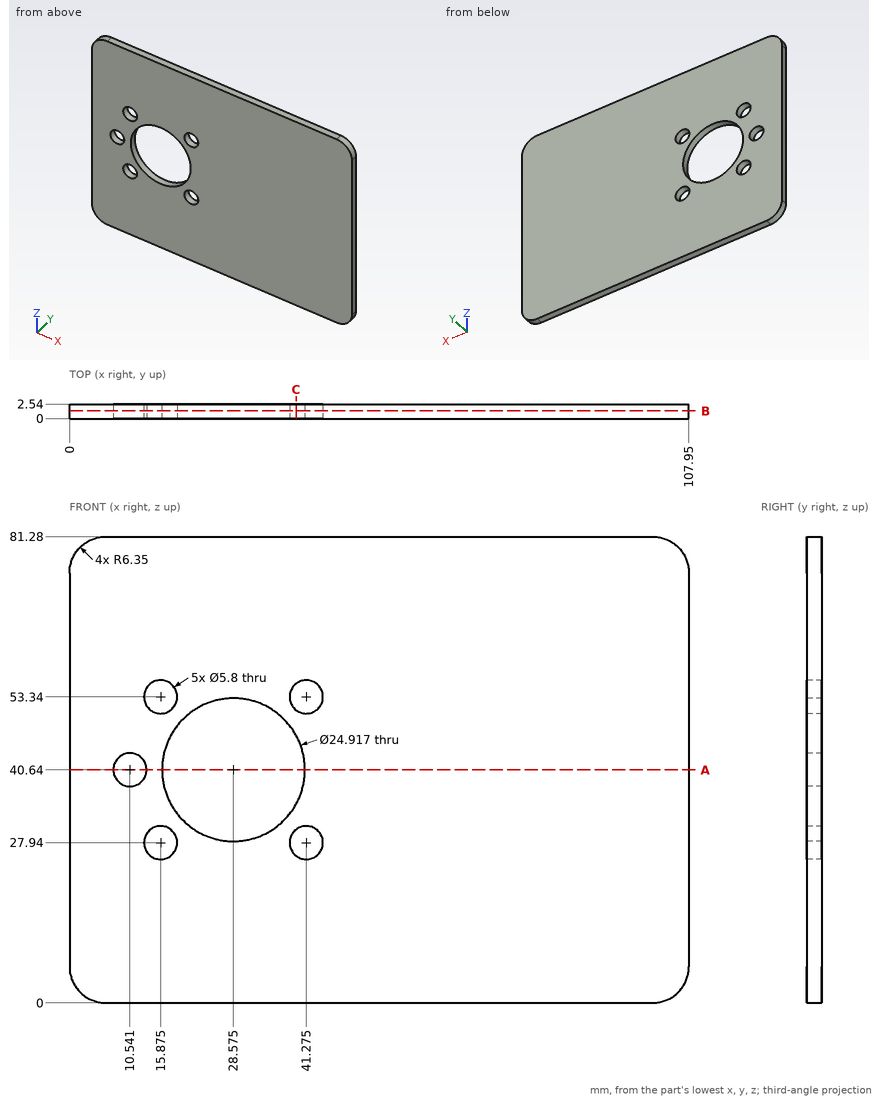
Source: three-view drawing plus pictorial views. Frame: mm from the lowest corner of the part. Give positions to 0.01 mm unless a question says otherwise; leave off trailing zeros. Order: outer loops, then holes, each group sorted by start corner. A loop starts at its lowest first (then second) coordinate and runs counter-clockwise, first axis right, second up. Notation, with made-up numbers: (3.5, -23) -> (49.5, -23) arc R17 cw to (49.5, 1) -> close; hole circle Ø3 at (2.5, 41). An arc over 180 degrees is marked (long way). Put each result on its own line as item: value.
Q1. Section C-C, the plane x = 39.5. Return loops of the section in (y, z).
Here are the results:
outline: (0, 0) -> (2.54, 0) -> (2.54, 25.65) -> (0, 25.65) -> close; (0, 30.23) -> (2.54, 30.23) -> (2.54, 34.65) -> (0, 34.65) -> close; (0, 46.63) -> (2.54, 46.63) -> (2.54, 51.05) -> (0, 51.05) -> close; (0, 55.63) -> (2.54, 55.63) -> (2.54, 81.28) -> (0, 81.28) -> close
Q2. Pin query (flat end, axial travel): pin 1 (3.5 mm diameter, centred on x = 41.275, z = 27.94, fed in from -Y). Return the tip coordinate at first contact, or that it passes through.
Here are the results:
pin 1: passes through
Q3. Section B-B, the plane y = 1.35. Count the separate pieces of the cut face and the enclosed holes in it, then the cut area to 3 significant figures.
Here are the results:
separate pieces: 1
enclosed holes: 6
area: 8,120 mm^2
Q4. Material intervals for L1, parallel to X at y = 0.7, z = 40.64; L2, parallel to X at y = 0.15, z = 27; L3, parallel to Z at x = 21, y = 2.2, sorted ascending.
Here are the results:
L1: x = 0 to 7.64, 13.44 to 16.12, 41.03 to 107.95
L2: x = 0 to 13.13, 18.62 to 38.53, 44.02 to 107.95
L3: z = 0 to 30.75, 50.53 to 81.28
Q5. Section A-A, the plane z = 40.64. Return loops of the section in (x, y).
Here are the results:
outline: (0, 0) -> (7.64, 0) -> (7.64, 2.54) -> (0, 2.54) -> close; (13.44, 0) -> (16.12, 0) -> (16.12, 2.54) -> (13.44, 2.54) -> close; (41.03, 0) -> (107.95, 0) -> (107.95, 2.54) -> (41.03, 2.54) -> close
